from build123d import *

# Parameters (mm, degrees)
F0_W            = 85
F0_H            = 80
F1_DEPTH        = 4
F3_DEPTH        = 12
F5_DEPTH        = 4
F6_R            = 5
F7_R            = 3
F8_R            = 6
F9_SIZE         = 1
F11_D           = 4
F11_CSINK_D     = 10
F11_CSINK_ANGLE = 82


with BuildPart() as f1:
    # F0 (on Top) → F1 (new body)
    with BuildSketch(Plane.XY):
        Rectangle(F0_W, F0_H)
    extrude(amount=F1_DEPTH)

    # F2 (on face) → F3 (join)
    with BuildSketch(Plane.XY.offset(4)):
        Polygon((-42.5, 40), (-42.5, -40), (-15, -40), (-15, -36), (-38.5, -36), (-38.5, 40), align=None)
        Polygon((42.5, 40), (38.5, 40), (38.5, -36), (15, -36), (15, -40), (42.5, -40), align=None)
    extrude(amount=F3_DEPTH)

    # F4 (on face) → F5 (join)
    with BuildSketch(Plane.XY.offset(16)):
        with BuildLine():
            Line((-42.5, 40), (-42.5, -40))
            Line((-42.5, -40), (-15, -40))
            Line((-15, -40), (-15, -36))
            Line((-15, -36), (-15, -30))
            Line((-15, -30), (-27.5, -30))
            ThreePointArc((-27.5, -30), (-31.0355339059, -28.5355339059), (-32.5, -25))
            Line((-32.5, -25), (-32.5, 40))
            Line((-32.5, 40), (-38.5, 40))
            Line((-38.5, 40), (-42.5, 40))
        make_face()
        with BuildLine():
            Line((38.5, 40), (32.5, 40))
            Line((32.5, 40), (32.5, -25))
            ThreePointArc((32.5, -25), (31.0355339059, -28.5355339059), (27.5, -30))
            Line((27.5, -30), (15, -30))
            Line((15, -30), (15, -36))
            Line((15, -36), (15, -40))
            Line((15, -40), (42.5, -40))
            Line((42.5, -40), (42.5, 40))
            Line((42.5, 40), (38.5, 40))
        make_face()
    extrude(amount=F5_DEPTH)

    # F6
    f6_edges = [f1.edges().sort_by_distance(p)[0] for p in [
        (-42.5, -40, 10),
        (42.5, -40, 10),
    ]]
    fillet(f6_edges, radius=F6_R)

    # F7
    f7_edges = [f1.edges().sort_by_distance(p)[0] for p in [
        (38.5, -36, 10),
        (-38.5, -36, 10),
    ]]
    fillet(f7_edges, radius=F7_R)

    # F8
    f8_edges = [f1.edges().sort_by_distance(p)[0] for p in [
        (-32.5, 40, 18),
        (32.5, 40, 18),
    ]]
    fillet(f8_edges, radius=F8_R)

    # F9
    f9_edges = [f1.edges().sort_by_distance(p)[0] for p in [
        (40.5, 40, 20),
        (38.5, 40, 18),
        (42.5, 40, 10),
        (38.5, 40, 10),
        (0, 40, 0),
        (0, 40, 4),
        (-42.5, 40, 10),
        (-38.5, 40, 10),
        (-40.5, 40, 20),
        (-38.5, 40, 18),
        (-26.25, -40, 20),
        (-37.5, -40, 10),
        (-15, -40, 12),
        (0, -40, 0),
        (0, -40, 4),
        (37.5, -40, 10),
        (15, -40, 12),
        (26.25, -40, 20),
        (41.035534, -38.535534, 0),
        (42.5, -35, 10),
        (41.035534, -38.535534, 20),
        (42.5, 2.5, 20),
        (42.5, 2.5, 0),
        (-41.035534, -38.535534, 20),
        (-42.5, -35, 10),
        (-41.035534, -38.535534, 0),
        (-42.5, 2.5, 20),
        (-42.5, 2.5, 0),
        (-25.25, -36, 4),
        (-37.62132, -35.12132, 4),
        (-15, -38, 4),
        (-38.5, 3.5, 4),
        (15, -38, 4),
        (38.5, 3.5, 4),
        (25.25, -36, 4),
        (37.62132, -35.12132, 4),
        (15, -36, 10),
        (15, -33, 16),
        (15, -30, 18),
        (15, -35, 20),
        (-15, -35, 20),
        (-15, -30, 18),
        (-15, -33, 16),
        (-15, -36, 10),
    ]]
    chamfer(f9_edges, length=F9_SIZE)

    # F11 (through all)
    with Locations(Plane.XY.offset(4)):
        with Locations((-20, 24), (20, 24), (0, -25)):
            CounterSinkHole(F11_D / 2, F11_CSINK_D / 2, counter_sink_angle=F11_CSINK_ANGLE)


solid = f1.part
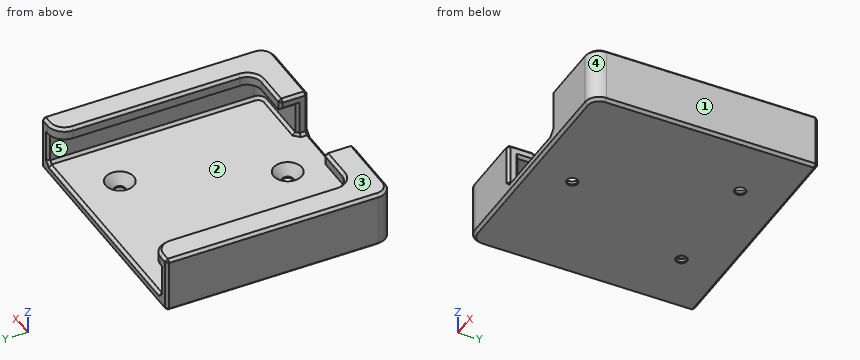
Here's how the part is built. I have some questions about the finished solid (model axes, mm). Face numbers are marked on the shaded views. A direction names the side the tool comes from. Coordinates: 2 decimals unless noted, no trailing zeros. Write each loop counter-clockwise with the first axis right and the second up, starting at its lowest first coordinate (ties: lowest second). Pieces come first, ordered by that corner, then holes.
1) Thinking about a two-plate mould opening in Z: for the marked faces 3, 4 and 5, which applies, +Z half, -Z half, draft (parallel to the pull), parting line (faces both ways), or undercut?
Filled in:
face 3: +Z half
face 4: draft
face 5: undercut
2) If we section it at B-B (x = 0): List the corners of the cut face in (y, z) for me, plus the area to 3 significant figures.
Filled in:
outline: (-40, 1) - (-39, 0) - (-27, 0) - (-27, 0.55) - (-30, 4) - (-39, 4) - (-40, 3) - close; (-23, 0) - (39, 0) - (40, 1) - (40, 3) - (39, 4) - (-20, 4) - (-23, 0.55) - close
area: 292 mm2
3) If we section it at A-A (y = 24): Count the separate pieces of the cut face and the enclosed holes in it, plus the area to 3 significant figures.
Filled in:
separate pieces: 3
enclosed holes: 0
area: 461 mm2
4) I'm going to push flat-ended pins straight in: pin 1 (3.5 mm diameter, centred on x = -28.5, z = 9.5, fed in from +Y); pin 2 (1.5 mm diameter, centred on x = -23.5, z = 17.5, fed in from +Y); pin 3 (3 mm diameter, centred on x = 14, y = 7.5, fed in from -Z); pin 4 (6.5 mm diameter, centred on x = 0, y = -25, fed in from +Z). Where does each tip first touch, or does it pass through?
Filled in:
pin 1: stops at y = -36
pin 2: stops at y = -30
pin 3: stops at z = 0
pin 4: stops at z = 1.99
5) Which directions (+Z, -Z, +X, -X, +Y, -Y) give clear straight access to the entire face, cutting with the end or side of a thin tool? Please do the marked faces 1 and 2.
Filled in:
face 1: +Z, -Z, +X, +Y, -Y
face 2: +Y
6) If we section it at C-C (z = 10.5): List the corners of the cut face in (x, y) for me, plus the area to 3 significant figures.
Filled in:
outline: (-42.5, -35) arc R5 ccw to (-37.5, -40) - (-16, -40) - (-15, -39) - (-15, -37) - (-16, -36) - (-35.5, -36) arc R3 cw to (-38.5, -33) - (-38.5, 39) - (-39.5, 40) - (-41.5, 40) - (-42.5, 39) - close; (15, -39) - (16, -40) - (37.5, -40) arc R5 ccw to (42.5, -35) - (42.5, 39) - (41.5, 40) - (39.5, 40) - (38.5, 39) - (38.5, -33) arc R3 cw to (35.5, -36) - (16, -36) - (15, -37) - close
area: 817 mm2
7) If we section it at D-D (y = -10.5): List the corners of the cut face in (x, z) for me.
Filled in:
outline: (-42.5, 1) - (-41.5, 0) - (41.5, 0) - (42.5, 1) - (42.5, 19) - (41.5, 20) - (33.5, 20) - (32.5, 19) - (32.5, 16) - (38.5, 16) - (38.5, 5) - (37.5, 4) - (-37.5, 4) - (-38.5, 5) - (-38.5, 16) - (-32.5, 16) - (-32.5, 19) - (-33.5, 20) - (-41.5, 20) - (-42.5, 19) - close
8) If I drill on line 1 (X direction, y = 24, z = 0.25); line 2 (X direction, y = -11, z = 11.5); line 3 (Z direction, x = -36, y = -8.5), over which ranges is the centre line in solid material (lowest first)?
Filled in:
line 1: x = -41.75 to -22, -18 to 18, 22 to 41.75
line 2: x = -42.5 to -38.5, 38.5 to 42.5
line 3: z = 0 to 4, 16 to 20
